The model under review builds one solid part; all positions refer to its coordinate system, in mm. Face numbers are marked on the shaded views. A direction names the side the tool comes from. Round coordinates to 2 decimals unless told otherwise and drop trailing zeros. Write each loop counter-clockwise with the first axis right and the second up, starting at its lowest first coordinate (ties: lowest second). Pieces come first, ordered by that corner, then holes. Notation, with made-up numbers: (-1, 65) -> (10, 65) arc R20 cw to (10, 85) -> close; hole circle Ø5 at (51, 43). An arc over 180 degrees is marked (long way). Answer in a Markdown table with one row per item. Add a question column.
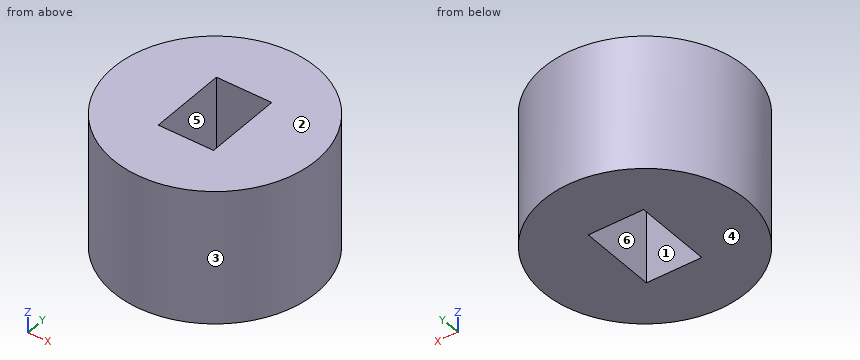
```python
from build123d import *

# Parameters (mm, degrees)
F0_W     = 38.5183766484
F0_H     = 50.980206579
F2_W     = 20.9750365466
F2_H     = 29.5896790922
F3_DEPTH = 50.981206579


with BuildPart() as f1:
    # F0 (on Right) → F1 (revolve)
    with BuildSketch(Plane.YZ):
        with Locations((-19.2591883242, 25.4901032895)):
            Rectangle(F0_W, F0_H)
    revolve(axis=Axis((0, 0, 25.4901032895), (0, 0, 1)))

    # F2 (on face) → F3 (cut, through all)
    with BuildSketch(Plane.XY.offset(50.980206579)):
        Rectangle(F2_W, F2_H)
    extrude(amount=-F3_DEPTH, mode=Mode.SUBTRACT)


solid = f1.part
```
1. Tool access review of the marked faces 1 and 2: name each direction out of +Z, -Z, +X, -X, +Y, -Y from which nothing blocks a thin tool from reaching the whole face with its end or side.
2. Add section C-C on z = 36.5. Write out the cut boundary in (x, y).
3. For L1, parallel to Y at x = -7, z = 34; L2, parallel to X at y = 13.5, z = 46.5; L3, parallel to X at y = 3, z = 16, list the stretches that pass through material, from the lowest coordinate up.
4. Add section B-B on y = 0. Write out the cut boundary in (x, z), plus the area to 3 significant figures.
5. Add section D-D on x = -19. Write out the cut boundary in (y, z), plus the area to 3 significant figures.
6. Mouldability with a two-part tool opening along Y and no side actions: class the marked faces 3, 4, 5 and 6 as pulls with the +Y half, pulls with the -Y half, needs draft (parallel to the pull), parting line crosses it, or undercut.
7. Insertion check: pin 1 Ø6 at (x, z) = (19.5, 15.5) entering from -Y; pin 2 Ø6 at (x, z) = (4.5, 36) entering from +Y; pin 3 Ø4 at (y, z) = (10, 19) entering from +X. Each pin has a flat end and moves straight along its axis. Give the tip position at first contact, or say it passes through.
8. Add section A-A on x = 0. Write out the cut boundary in (y, z).
Filled in:
| question | item | result |
|---|---|---|
| 1 | face 1 | +Z, -Z |
| 1 | face 2 | +Z, +X, -X, +Y, -Y |
| 2 | outline | circle Ø77.04 at (0, 0); hole (-10.49, -14.79) -> (10.49, -14.79) -> (10.49, 14.79) -> (-10.49, 14.79) -> close |
| 3 | L1 | -37.88 to -14.79, 14.79 to 37.88 |
| 3 | L2 | -36.08 to -10.49, 10.49 to 36.08 |
| 3 | L3 | -38.4 to -10.49, 10.49 to 38.4 |
| 4 | outline | (-38.52, 0) -> (-10.49, 0) -> (-10.49, 50.98) -> (-38.52, 50.98) -> close; (10.49, 0) -> (38.52, 0) -> (38.52, 50.98) -> (10.49, 50.98) -> close |
| 4 | area | 2,860 mm² |
| 5 | outline | (-33.51, 0) -> (33.51, 0) -> (33.51, 50.98) -> (-33.51, 50.98) -> close |
| 5 | area | 3,420 mm² |
| 6 | face 3 | parting line crosses it |
| 6 | face 4 | needs draft |
| 6 | face 5 | undercut |
| 6 | face 6 | undercut |
| 7 | pin 1 | y = -34.81 |
| 7 | pin 2 | y = 38.49 |
| 7 | pin 3 | x = 37.68 |
| 8 | outline | (-38.52, 0) -> (-14.79, 0) -> (-14.79, 50.98) -> (-38.52, 50.98) -> close; (14.79, 0) -> (38.52, 0) -> (38.52, 50.98) -> (14.79, 50.98) -> close |
